from build123d import *

# Parameters (mm, degrees)
SKETCH1_R           = 1.5
BOSS_EXTRUDE1_DEPTH = 22.5
SKETCH2_W           = 3.83
SKETCH2_H           = 8.7
SKETCH2_W_2         = 8
SKETCH2_H_2         = 30.35
SKETCH2_W_3         = 13.1
SKETCH2_H_3         = 15
CUT_EXTRUDE1_DEPTH  = 55.757415023
BOSS_EXTRUDE2_START = 6.33
SKETCH3_W           = 77.56
SKETCH3_H           = 24.7
BOSS_EXTRUDE2_DEPTH = 6.33
CHAMFER1_SIZE       = 2.5
CHAMFER2_SIZE       = 1.5
BOSS_EXTRUDE3_DEPTH = 3.31
SKETCH5_R           = 3
BOSS_EXTRUDE4_DEPTH = 2.4
FILLET1_R           = 0.5
SKETCH6_R           = 1.25
CUT_EXTRUDE2_DEPTH  = 10


with BuildPart() as part:
    # Sketch1 → Boss-Extrude1 (new, symmetric)
    with BuildSketch(Plane.XY):
        with BuildLine():
            Line((-45.5, 3.83), (45.5, 3.83))
            ThreePointArc((45.5, 3.83), (49.33, 0), (45.5, -3.83))
            Line((45.5, -3.83), (-45.5, -3.83))
            ThreePointArc((-45.5, -3.83), (-49.33, 0), (-45.5, 3.83))
        make_face()
        with Locations(Location((-45.5, 0, 0), (0, 0, 180))):
            Circle(SKETCH1_R, mode=Mode.SUBTRACT)
        with Locations(Location((45.5, 0, 0), (0, 0, 180))):
            Circle(SKETCH1_R, mode=Mode.SUBTRACT)
    extrude(amount=BOSS_EXTRUDE1_DEPTH, both=True)

    # Sketch2 → Cut-Extrude1 (cut, through all)
    with BuildSketch(Plane(origin=(0, 3.83, 0), x_dir=(1, 0, 0), z_dir=(0, 1, 0))):
        Polygon((-10.33, 13.8), (45.5, 13.8), (45.5, 22.5), (-33.33, 22.5), align=None)
        Polygon((41.67, -13.8), (-41.67, -22.5), (45.5, -22.5), (45.5, -13.8), align=None)
        with Locations((47.415, -18.15)):
            Rectangle(SKETCH2_W, SKETCH2_H)
        with Locations((47.415, 18.15)):
            Rectangle(SKETCH2_W, SKETCH2_H)
        with BuildLine():
            Line((-6.43, 7.5), (-28.43, 7.5))
            ThreePointArc((-28.43, 7.5), (-31.258427125, 6.328427125), (-32.43, 3.5))
            Line((-32.43, 3.5), (-32.43, -3.5))
            ThreePointArc((-32.43, -3.5), (-31.258427125, -6.328427125), (-28.43, -7.5))
            Line((-28.43, -7.5), (-6.43, -7.5))
            ThreePointArc((-6.43, -7.5), (-3.601572875, -6.328427125), (-2.43, -3.5))
            Line((-2.43, -3.5), (-2.43, 3.5))
            ThreePointArc((-2.43, 3.5), (-3.601572875, 6.328427125), (-6.43, 7.5))
        make_face()
        with BuildLine():
            Line((25.23, 7.5), (7.23, 7.5))
            ThreePointArc((7.23, 7.5), (4.401572875, 6.328427125), (3.23, 3.5))
            Line((3.23, 3.5), (3.23, -3.5))
            ThreePointArc((3.23, -3.5), (4.401572875, -6.328427125), (7.23, -7.5))
            Line((7.23, -7.5), (25.23, -7.5))
            ThreePointArc((25.23, -7.5), (28.058427125, -6.328427125), (29.23, -3.5))
            Line((29.23, -3.5), (29.23, 3.5))
            ThreePointArc((29.23, 3.5), (28.058427125, 6.328427125), (25.23, 7.5))
        make_face()
        with Locations((-45.33, 0)):
            Rectangle(SKETCH2_W_2, SKETCH2_H_2)
        with Locations((42.78, 0)):
            Rectangle(SKETCH2_W_3, SKETCH2_H_3)
    extrude(amount=-CUT_EXTRUDE1_DEPTH, mode=Mode.SUBTRACT)

    # Sketch3 → Boss-Extrude2 (add)
    with BuildSketch(Plane(origin=(0, 0, 0), x_dir=(1, 0, 0), z_dir=(0, 1, 0)).offset(BOSS_EXTRUDE2_START)):
        with Locations((-2.55, 0)):
            Rectangle(SKETCH3_W, SKETCH3_H)
        with BuildLine():
            ThreePointArc((3.23, -3.5), (4.401572875, -6.328427125), (7.23, -7.5))
            Line((7.23, -7.5), (25.23, -7.5))
            ThreePointArc((25.23, -7.5), (28.058427125, -6.328427125), (29.23, -3.5))
            Line((29.23, -3.5), (29.23, 3.5))
            ThreePointArc((29.23, 3.5), (28.058427125, 6.328427125), (25.23, 7.5))
            Line((25.23, 7.5), (7.23, 7.5))
            ThreePointArc((7.23, 7.5), (4.401572875, 6.328427125), (3.23, 3.5))
            Line((3.23, 3.5), (3.23, -3.5))
        make_face(mode=Mode.SUBTRACT)
        with BuildLine():
            ThreePointArc((-32.43, -3.5), (-31.258427125, -6.328427125), (-28.43, -7.5))
            Line((-28.43, -7.5), (-6.43, -7.5))
            ThreePointArc((-6.43, -7.5), (-3.601572875, -6.328427125), (-2.43, -3.5))
            Line((-2.43, -3.5), (-2.43, 3.5))
            ThreePointArc((-2.43, 3.5), (-3.601572875, 6.328427125), (-6.43, 7.5))
            Line((-6.43, 7.5), (-28.43, 7.5))
            ThreePointArc((-28.43, 7.5), (-31.258427125, 6.328427125), (-32.43, 3.5))
            Line((-32.43, 3.5), (-32.43, -3.5))
        make_face(mode=Mode.SUBTRACT)
    extrude(amount=-BOSS_EXTRUDE2_DEPTH)

    # Chamfer1
    chamfer1_edges = [part.edges().sort_by_distance(p)[0] for p in [
        (36.23, 6.33, 0),
        (-41.33, 6.33, 0),
    ]]
    chamfer(chamfer1_edges, length=CHAMFER1_SIZE)

    # Chamfer2
    chamfer2_edges = [part.edges().sort_by_distance(p)[0] for p in [
        (-2.55, 6.33, 12.35),
        (-2.55, 6.33, -12.35),
    ]]
    chamfer(chamfer2_edges, length=CHAMFER2_SIZE)

    # Sketch4 → Boss-Extrude3 (add)
    with BuildSketch(Plane(origin=(0, 0, -13.8), x_dir=(-1, 0, 0), z_dir=(0, 0, -1))):
        with BuildLine():
            Line((21.5, -2.93), (-12.5, -2.93))
            ThreePointArc((-12.5, -2.93), (-15.43, 0), (-12.5, 2.93))
            Line((-12.5, 2.93), (21.5, 2.93))
            ThreePointArc((21.5, 2.93), (24.43, 0), (21.5, -2.93))
        make_face()
    extrude(amount=BOSS_EXTRUDE3_DEPTH)

    # Sketch5 → Boss-Extrude4 (add)
    with BuildSketch(Plane(origin=(0, 0, -17.11), x_dir=(-1, 0, 0), z_dir=(0, 0, -1))):
        with Locations(Location((21.5, 0, 0), (0, 0, 216.247045378))):
            Circle(SKETCH5_R)
    extrude(amount=BOSS_EXTRUDE4_DEPTH)

    # Fillet1
    fillet1_edges = [part.edges().sort_by_distance(p)[0] for p in [
        (-23.919425287, 1.773804183, -19.51),
    ]]
    fillet(fillet1_edges, radius=FILLET1_R)

    # Sketch6 → Cut-Extrude2 (cut)
    with BuildSketch(Plane(origin=(0, 0, -19.51), x_dir=(-1, 0, 0), z_dir=(0, 0, -1))):
        with Locations((21.5, 0)):
            Circle(SKETCH6_R)
        with Locations((9.1, 0)):
            Circle(SKETCH6_R)
        with Locations((1.9, 0)):
            Circle(SKETCH6_R)
        with Locations((-5.3, 0)):
            Circle(SKETCH6_R)
        with Locations((-12.5, 0)):
            Circle(SKETCH6_R)
        with Locations((-8.9, 0)):
            Circle(SKETCH6_R)
    extrude(amount=-CUT_EXTRUDE2_DEPTH, mode=Mode.SUBTRACT)


solid = part.part
Can you work these out from the model? Positions are in its coordinate system, mm. A direction names the side the tool comes from. Give positions to 0.01 mm unless a question says otherwise; leave off trailing zeros. Loops run counter-clockwise (first coordinate to the right, second up) from the corner with the lowest first, then second, coordinate; pieces in that order, holes last. Notation, with made-up numbers: (-34, 27) -> (21, 27) arc R11 cw to (21, 32) -> close; hole circle Ø8 at (-9, 62.25). An arc over 180 degrees is marked (long way). Return JSON: item names as keys, results as strings.
Q1. I need wall thicknesses on probe 1 along Y at (x, z) = (8.9, -13.5); probe 2 along X at (y, z) = (5, 3); probe 3 along X at (y, z) = (3.75, -4). Which ranges of each line are inside material? Lowest first, please.
Checks:
{"probe 1": "y = -3.83 to -1.25, 1.25 to 3.83", "probe 2": "x = -40.16 to -32.43, -2.43 to 3.23, 29.23 to 35.06", "probe 3": "x = -41.33 to -32.4, -2.46 to 3.26, 29.2 to 36.23"}
Q2. I want a section at A-A, the plane z = 8.5. List the corners of the cut face in (x, y) for me, then the cut area to 3 significant figures.
Checks:
{"outline": "(-41.33, -3.83) -> (45.5, -3.83) arc R3.83 ccw to (45.5, 3.83) -> (36.23, 3.83) -> (33.73, 6.33) -> (-38.83, 6.33) -> (-41.33, 3.83) -> close; hole circle Ø3 at (45.5, 0)", "area": "869 mm2"}
Q3. We'd pull the mould along X, two halves only. Please class faces 1 (the face through (-41.33, 0, 0)), 2 (the face through (4.11, 0.38, -13.36)), 3 (the face through (15.43, -0.06, -15.43)): released by +X, released by -X, zero draft, split by the parting line, or undercut.
Checks:
{"face 1": "released by -X", "face 2": "undercut", "face 3": "released by +X"}
Q4. For pin 1 Ø4 at (x, y) = (17, 0) entering from +Z; pin 2 Ø3.5 at (y, z) = (2, -1.5) entering from -X; pin 3 Ø2.5 at (x, y) = (45, -1.5) entering from -Z, each with a flat end and sliding along its axis, tell me the tip position at first contact or that it passes through.
Checks:
{"pin 1": "stops at z = 16.58", "pin 2": "stops at x = -41.33", "pin 3": "stops at z = -13.8"}
Q5. On a 3-axis mill with a long thin cutter (end or side, diameter ignored), from which of +Z, -Z, +X, -X, +Y, -Y can I reach the whole of each face in a straight line? I mean faces 4 (the face through (47, 0, -11)), 5 (the face through (13, 0, -9.51)), 6 (the face through (-14, 3.83, -15)), 7 (the face through (-49.33, -0.08, -18.79)), 8 (the face through (-3.633, 1.321, 6.359)). Say none if no direction works.
Checks:
{"face 4": "+Z, -Z", "face 5": "-Z", "face 6": "-Z, +X, +Y", "face 7": "+Z, -Z, -X", "face 8": "+Y, -Y"}
Q6. I want a section at C-C, the plane x = 8.9. List the corners of the cut face in (y, z) for me, then the cut area to 3 significant figures.
Checks:
{"outline": "(-3.83, -13.8) -> (-2.93, -13.8) -> (-2.93, -17.11) -> (-1.25, -17.11) -> (-1.25, -9.51) -> (1.25, -9.51) -> (1.25, -17.11) -> (2.93, -17.11) -> (2.93, -13.8) -> (3.83, -13.8) -> (3.83, -12.35) -> (4.83, -12.35) -> (6.33, -10.85) -> (6.33, -7.5) -> (-3.83, -7.5) -> close; (-3.83, 7.5) -> (6.33, 7.5) -> (6.33, 10.85) -> (4.83, 12.35) -> (3.83, 12.35) -> (3.83, 17.22) -> (-3.83, 17.22) -> close", "area": "145 mm2"}
Q7. I want a section at D-D, the plane y = 0. Count the separate pieces of the cut face and the enclosed holes in it, then the cut area to 3 significant figures.
Checks:
{"separate pieces": "5", "enclosed holes": "2", "area": "2,050 mm2"}
Q8. I want a section at B-B, the plane z = 0.5. List the corners of the cut face in (x, y) for me.
Checks:
{"outline": "(-41.33, -3.83) -> (-32.43, -3.83) -> (-32.43, 6.33) -> (-38.83, 6.33) -> (-41.33, 3.83) -> close; (-2.43, -3.83) -> (3.23, -3.83) -> (3.23, 6.33) -> (-2.43, 6.33) -> close; (29.23, -3.83) -> (36.23, -3.83) -> (36.23, 3.83) -> (33.73, 6.33) -> (29.23, 6.33) -> close"}
